Geometry check sheet. Reference: drawing and pictorial views, mm from the part's lowest x, y, z. Round coordinates to 2 decimals unless told otherwise and drop trailing zeros. Order: outer loops, then holes, each group sorted by start corner. A loop starts at its lowest first (then second) coordinate and runs counter-clockwise, first axis right, second up. Notation, with made-up numbers: (-6, -24.75) -> (21, -24.75) arc R9 cw to (21, -8.75) -> close; hole circle Ø3 at (3.5, -30.75). An arc over 180 degrees is marked (long way). Put each result on its own line as item: value.
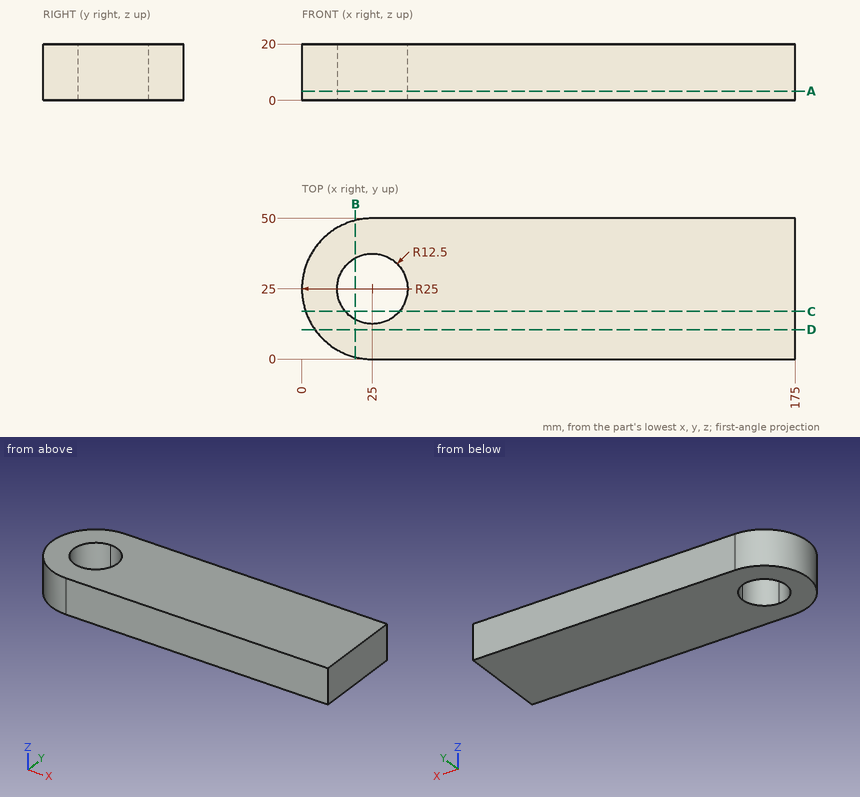
Item 1: Sectioned sample at C-C, the plane y = 17. Record the boundary of the cut face in (x, z).
Geometry check:
outline: (1.31, 0) -> (15.4, 0) -> (15.4, 20) -> (1.31, 20) -> close; (34.6, 0) -> (175, 0) -> (175, 20) -> (34.6, 20) -> close
Item 2: Material ranges on line 1 along Y through (x, z) = (23, 17.75); line 2 along X through (y, z) = (35.5, 8.25); line 3 along X through (y, z) = (18.5, 14), recorded low to high.
Geometry check:
line 1: 0.08 to 12.66, 37.34 to 49.92
line 2: 2.31 to 18.22, 31.78 to 175
line 3: 0.86 to 14.32, 35.68 to 175
Item 3: Depth check by flat-ended pin: pin 1 Ø4 at (x, z) = (21, 5) entering from +Y; pin 2 Ø4 at (y, z) = (43, 8) entering from -X; pin 3 Ø5 at (y, z) = (13, 6) entering from -X. Enter the tip coordinate at first touch or a pass-through.
Geometry check:
pin 1: y = 49.92
pin 2: x = 5.79
pin 3: x = 1.88
Item 4: Sectioned sample at B-B, the plane x = 19. Record the boundary of the cut face in (y, z).
Geometry check:
outline: (0.73, 0) -> (14.03, 0) -> (14.03, 20) -> (0.73, 20) -> close; (35.97, 0) -> (49.27, 0) -> (49.27, 20) -> (35.97, 20) -> close
Item 5: Sectioned sample at D-D, the plane y = 10.5. Record the boundary of the cut face in (x, z).
Geometry check:
outline: (4.63, 0) -> (175, 0) -> (175, 20) -> (4.63, 20) -> close
Item 6: Sectioned sample at A-A, the plane z = 3.25. Record the boundary of the cut face in (x, y).
Geometry check:
outline: (25, 0) -> (175, 0) -> (175, 50) -> (25, 50) arc R25 ccw to start; hole circle Ø25 at (25, 25)
